from build123d import *

# Parameters (mm, degrees)
F0_R     = 9.5631
F1_DEPTH = 2.5
F2_R     = 8.9162314004
F2_R_2   = 7.9162314004
F3_DEPTH = 0.5
F4_R     = 4
F5_DEPTH = 3.5
F6_R     = 1.2071067812
F7_R     = 2
F8_DEPTH = 3
F9_R     = 0.7966904756


with BuildPart() as f1:
    # F0 (on Top) → F1 (new body)
    with BuildSketch(Plane.XY):
        Circle(F0_R)
    extrude(amount=F1_DEPTH)

    # F2 (on face) → F3 (cut)
    with BuildSketch(Plane.XY.offset(2.5)):
        Circle(F2_R)
        Circle(F2_R_2, mode=Mode.SUBTRACT)
        Polygon((1.8036346717, 5.9258921407), (-2.7067440096, 5.9258921407), (-2.7067440096, 4.4258921407), (-1.8036346717, 4.4258921407), (-1.8036346717, 3.1822535675), (-5.7792644948, 3.1822535675), (-5.7792644948, -4.3527372181), (-4.1694175287, -4.3527372181), (-4.1694175287, -2.3218090646), (-3.4134816378, -2.3218090646), (-3.4134816378, 0), (-1.8036346717, 0), (-2.0609125495, -6.6612055525), (0, -6.6612055525), (2.0609125495, -6.6612055525), (1.8036346717, 0), (3.4134816378, 0), (3.4134816378, -2.3218090646), (4.1694175287, -2.3218090646), (4.1694175287, -4.3527372181), (5.7792644948, -4.3527372181), (5.7792644948, 3.1822535675), (1.8036346717, 3.1822535675), align=None)
    extrude(amount=-F3_DEPTH, mode=Mode.SUBTRACT)

    # F4 (on face) → F5 (join)
    with BuildSketch(Plane(origin=(0, 0, 0), x_dir=(1, 0, 0), z_dir=(0, 0, -1))):
        Circle(F4_R)
    extrude(amount=F5_DEPTH)

    # F6
    f6_edges = [f1.edges().sort_by_distance(p)[0] for p in [
        (-9.5631, 0, 0),
    ]]
    fillet(f6_edges, radius=F6_R)

    # F7 (on face) → F8 (cut)
    with BuildSketch(Plane(origin=(0, 0, -3.5), x_dir=(1, 0, 0), z_dir=(0, 0, -1))):
        Circle(F7_R)
    extrude(amount=-F8_DEPTH, mode=Mode.SUBTRACT)

    # F9
    f9_edges = [f1.edges().sort_by_distance(p)[0] for p in [
        (-4, 0, -3.5),
    ]]
    fillet(f9_edges, radius=F9_R)


solid = f1.part
Here's how the part is built. I have some questions about the finished solid (model axes, mm). A direction names the side the tool comes from. Give positions to 0.01 mm unless a question says otherwise; leave off trailing zeros. Loops run counter-clockwise (first coordinate to the right, second up) from the corner with the lowest first, then second, coordinate; pieces in that order, holes last. Notation, with made-up numbers: (48, 76.25) -> (102, 76.25) arc R23 cw to (102, 114.25) -> close; hole circle Ø5 at (-15, -0.5). An arc over 180 degrees is marked (long way). One line per item, written item: value.
Q1. I'm going to push flat-ended pins straight in: pin 1 Ø0.6 at (x, z) = (-2.5, 2) entering from +Y; pin 2 Ø0.6 at (x, z) = (4.5, 2.5) entering from -Y; pin 3 Ø0.6 at (y, z) = (-1, 2) entering from +X; pin 4 Ø1 at (y, z) = (-6.5, -1) entering from +X. Where does each tip first touch, or does it pass through?
Answers follow:
pin 1: y = 9.31
pin 2: y = -8.59
pin 3: x = 9.54
pin 4: through
Q2. On a 3-axis mill with a long thin cutter (end or side, diameter ignored), from which of +Z, -Z, +X, -X, +Y, -Y can I reach the whole of each face in a straight line? I mean faces 1 (the face through (2, 1, -3.5)), 2 (the face through (-0.867, 3.905, -1.333)), 3 (the face through (-1.4, 8, 2)). Say none if no direction works.
Answers follow:
face 1: -Z, +X, -X, +Y, -Y
face 2: -Z
face 3: +Z
Q3. Suppose I cut it at A-A on x = 0. Please give me the cut outline in (y, z).
Answers follow:
outline: (-9.56, 1.21) arc R1.21 ccw to (-8.36, 0) -> (-4, 0) -> (-4, -2.7) arc R0.8 ccw to (-3.2, -3.5) -> (-2, -3.5) -> (-2, -0.5) -> (2, -0.5) -> (2, -3.5) -> (3.2, -3.5) arc R0.8 ccw to (4, -2.7) -> (4, 0) -> (8.36, 0) arc R1.21 ccw to (9.56, 1.21) -> (9.56, 2.5) -> (8.92, 2.5) -> (8.92, 2) -> (7.92, 2) -> (7.92, 2.5) -> (5.93, 2.5) -> (5.93, 2) -> (-6.66, 2) -> (-6.66, 2.5) -> (-7.92, 2.5) -> (-7.92, 2) -> (-8.92, 2) -> (-8.92, 2.5) -> (-9.56, 2.5) -> close
Q4. If I drill on line 1 along Y through (x, z) = (0, 2.4); line 2 along X through (y, z) = (0, -1.65); line 3 along Y through (x, z) = (0, -2.8), over which ranges is the centre line in solid material (lowest first)?
Answers follow:
line 1: -9.56 to -8.92, -7.92 to -6.66, 5.93 to 7.92, 8.92 to 9.56
line 2: -4 to -2, 2 to 4
line 3: -3.99 to -2, 2 to 3.99
Q5. Suppose I cut it at B-B on z = 0.95. Please give me the cut outline in (x, y), then the cut area to 3 significant figures.
Answers follow:
outline: circle Ø19.07 at (0, 0)
area: 286 mm^2
Q6. We'd pull the mould along X, two halves only. Please class faces 4 (the face through (3, -2, 2.5)), 5 (the face through (9.121, 2.872, 1.845)), 6 (the face through (-1.933, -8.704, 2.254)): pulls with the +X half, pulls with the -X half, needs draft (parallel to the pull), parting line crosses it, or undercut.
Answers follow:
face 4: needs draft
face 5: parting line crosses it
face 6: undercut
